Check sheet for the modelled part. Datum: model origin and axes. Units: mm. A direction names the side the tool comes from. Give positions to 0.01 mm unless a question says otherwise; leave off trailing zeros. Loops run counter-clockwise (first coordinate to the right, second up) from the corner with the lowest first, then second, coordinate; pieces in that order, holes last. Notation, with made-up numbers: (70, 38.25) - (119, 38.25) arc R20 ccw to (119, 64.25) - close; hole circle Ø3 at (50, 68.5). An arc over 180 degrees is marked (long way). Answer in a Markdown table with one row per item. Add a question column.
(1) Sectioned sample at D-D on y = 12.75. State how many separate pieces and enclosed holes the cut face has, then the cut area to 3 significant figures.
(2) Sectioned sample at C-C on x = -30.5. Enter the section's corners in (y, z).
(3) Thickness scan on L1, parallel to Z at x = 6.5, y = 11; L2, parallel to X at y = 14.25, z = 154.5; L3, parallel to Z at x = -19.5, y = 4. Record the ranges inside material, lowest first.
(4) Set-up check for faces 1 (the face through (0, 5, 128)), 2 (the face through (18.546, 10, 119)), 3 (the face through (8.945, 10.647, 149.074)), 4 (the face through (-0.31, 16.57, 128.29)): record each of +Z, -Z, +X, -X, +Y, -Y from which the full face is reachable in a straight line by a thin tool's end or side.
(5) Sectioned sample at A-A on x = 16. Enter the section's corners in (y, z).
(6) Draft check along Z on faces 5 (the face through (15.861, 11.11, 129.727)), 6 (the face through (29.046, 9.39, 161.315)), 7 (the face through (-22.925, 15, 143)). Enter one of: released by +Z, released by -Z, zero draft, split by the parting line, or undercut.
(7) Go/stop test with flat-tipped pins: P1, Ø1.5, axis at y = 11.5, z = 119.5, coming from the +X side; P2, Ø8, axis at x = -24, z = 135, coming from the +Y side; P3, Ø3, axis at y = 9.5, z = 135, coming from the +X side. Record where each tip stops, or that it passes through.
(8) Sectioned sample at B-B on z = 165. Enter the section's corners in (x, y), then the cut area to 3 significant figures.
from build123d import *

# Parameters (mm, degrees)
SKETCH2_W                       = 140.99708831
SKETCH2_H                       = 23.719356628
BOSS_EXTRUDE1_DEPTH             = 40
CUT_EXTRUDE1_DEPTH              = 229.787753821
BOSS_EXTRUDE2_DEPTH             = 16
CUT_EXTRUDE2_START              = -9
CUT_EXTRUDE2_DEPTH              = 9
FILLET1_R                       = 7
CUT_EXTRUDE3_DEPTH              = 194.183131235
CUT_EXTRUDE3_DEPTH_BACK         = 194.183131235
CUT_EXTRUDE4_DEPTH              = 194.497622924
BOSS_EXTRUDE4_REACH             = 195.183
SKETCH11_W                      = 140.99708831
SKETCH11_H                      = 8.5
BOSS_EXTRUDE4_DIRECTION_2_REACH = 195.183
SKETCH14_R                      = 0.7
CUT_EXTRUDE6_DEPTH              = 4
CUT_EXTRUDE7_DEPTH              = 202.370124673


with BuildPart() as part:
    # Sketch2 → Boss-Extrude1 (new body)
    with BuildSketch(Plane.XY.offset(138.608649029)):
        with Locations((-0.054079367, 11.859678314)):
            Rectangle(SKETCH2_W, SKETCH2_H)
    extrude(amount=BOSS_EXTRUDE1_DEPTH)

    # Sketch3 → Cut-Extrude1 (cut, through all)
    with BuildSketch(Plane.ZY.offset(70.552623522)):
        with BuildLine():
            Line((168.608649029, 23.719356628), (158.608649029, 23.719356628))
            Line((158.608649029, 23.719356628), (138.608649029, 23.719356628))
            Line((138.608649029, 23.719356628), (138.608649029, 5))
            ThreePointArc((138.608649029, 5), (156.289247948, 10.063699068), (168.608649029, 23.719356628))
        make_face()
    extrude(amount=-CUT_EXTRUDE1_DEPTH, mode=Mode.SUBTRACT)

    # Sketch4 → Boss-Extrude2 (add)
    with BuildSketch(Plane(origin=(0, 5, 0), x_dir=(1, 0, 0), z_dir=(0, 1, 0))):
        with BuildLine():
            Line((-22.924910668, -128.108649029), (-22.924910668, -168.608649029))
            Line((-22.924910668, -168.608649029), (-0.054079367, -168.608649029))
            Line((-0.054079367, -168.608649029), (22.816751934, -168.608649029))
            Line((22.816751934, -168.608649029), (22.816751934, -128.108649029))
            ThreePointArc((22.816751934, -128.108649029), (14.187021689, -127.958138772), (18.545920633, -120.508649029))
            Line((18.545920633, -120.508649029), (18.545920633, -117.508649029))
            Line((18.545920633, -117.508649029), (-18.654079367, -117.508649029))
            Line((-18.654079367, -117.508649029), (-18.654079367, -120.508649029))
            ThreePointArc((-18.654079367, -120.508649029), (-15.118545461, -121.973115123), (-13.654079367, -125.508649029))
            ThreePointArc((-13.654079367, -125.508649029), (-17.303923173, -130.322906838), (-22.924910668, -128.108649029))
        make_face()
    extrude(amount=BOSS_EXTRUDE2_DEPTH)

    # Sketch6 → Cut-Extrude2 (cut)
    with BuildSketch(Plane(origin=(0, 23.719356628, 0), x_dir=(1, 0, 0), z_dir=(0, 1, 0)).offset(CUT_EXTRUDE2_START)):
        with BuildLine():
            ThreePointArc((-18.654079367, -120.508649029), (-13.654079367, -125.508649029), (-18.654079367, -130.508649029))
            Line((-18.654079367, -130.508649029), (18.545920633, -130.508649029))
            ThreePointArc((18.545920633, -130.508649029), (13.545920633, -125.508649029), (18.545920633, -120.508649029))
            Line((18.545920633, -120.508649029), (18.545920633, -117.508649029))
            Line((18.545920633, -117.508649029), (-18.654079367, -117.508649029))
            Line((-18.654079367, -117.508649029), (-18.654079367, -120.508649029))
        make_face()
    extrude(amount=CUT_EXTRUDE2_DEPTH, mode=Mode.SUBTRACT)

    # Fillet1
    # the kernel refuses this fillet: 7 mm, written as the material it adds along each edge
    with BuildSketch(Plane(origin=(-36.061428038, 14.719356628, 130.508649029), x_dir=(0, 1, 0), z_dir=(1, 0, 0))) as fillet1_piece_1_section:
        with BuildLine():
            CenterArc((7, -6.962939469), FILLET1_R, 95.898427251, 84.101572749)
            Line((0, -6.962939469), (0, 0))
            Line((0, 0), (6.280643372, 0))
        make_face()
    fillet1_piece_1 = extrude(amount=72.014697343, mode=Mode.PRIVATE)
    fillet1_piece_1 = split(fillet1_piece_1, bisect_by=Plane(origin=(22.816751934, 16.511100944, 128.243610021), z_dir=(-1, 0, 0)), keep=Keep.TOP, mode=Mode.PRIVATE)
    fillet1_piece_1 = split(fillet1_piece_1, bisect_by=Plane(origin=(-22.924910668, 16.511100944, 128.243610021), z_dir=(1, 0, 0)), keep=Keep.TOP, mode=Mode.PRIVATE)
    fillet1_piece_1 = fillet1_piece_1 - Plane(origin=(18.545920633, 16.511100944, 125.508649029), x_dir=(0.854166260162501, 0, 0.5200000000000065), z_dir=(0, -1, 0)) * Cylinder(5, 172, mode=Mode.PRIVATE)
    fillet1_piece_1 = fillet1_piece_1 - Plane(origin=(-18.654079367, 16.511100944, 125.508649029), x_dir=(0, 0, -1), z_dir=(0, -1, 0)) * Cylinder(5, 172, mode=Mode.PRIVATE)
    add(fillet1_piece_1)

    # Sketch10 → Cut-Extrude3 (cut, two sides: drawn at the far end of the back side and taken through both)
    with BuildSketch(Plane(origin=(0, 21, 0), x_dir=(1, 0, 0), z_dir=(0, 1, 0)).offset(-CUT_EXTRUDE3_DEPTH_BACK)):
        with BuildLine():
            Line((-70.552623522, -168.608649029), (-70.552623522, -172.108649029))
            Line((-70.552623522, -172.108649029), (-56.424910668, -172.108649029))
            ThreePointArc((-56.424910668, -172.108649029), (-32.736833498, -162.296726199), (-22.924910668, -138.608649029))
            Line((-22.924910668, -138.608649029), (-70.552623522, -138.608649029))
            Line((-70.552623522, -138.608649029), (-70.552623522, -168.608649029))
        make_face()
        with BuildLine():
            ThreePointArc((22.816751934, -138.608649029), (32.628674764, -162.296726199), (56.316751934, -172.108649029))
            Line((56.316751934, -172.108649029), (70.444464788, -172.108649029))
            Line((70.444464788, -172.108649029), (70.444464788, -168.608649029))
            Line((70.444464788, -168.608649029), (70.444464788, -138.608649029))
            Line((70.444464788, -138.608649029), (22.816751934, -138.608649029))
        make_face()
    extrude(amount=CUT_EXTRUDE3_DEPTH + CUT_EXTRUDE3_DEPTH_BACK, mode=Mode.SUBTRACT)

    # Sketch12 → Cut-Extrude4 (cut, through all)
    with BuildSketch(Plane(origin=(0, 23.719356628, 0), x_dir=(1, 0, 0), z_dir=(0, 1, 0))):
        with BuildLine():
            ThreePointArc((39.183618102, -173.086260969), (47.517265008, -176.089564571), (56.316751934, -177.108649029))
            Line((56.316751934, -177.108649029), (70.444464788, -177.108649029))
            Line((70.444464788, -177.108649029), (70.444464788, -172.108649029))
            Line((70.444464788, -172.108649029), (56.316751934, -172.108649029))
            ThreePointArc((56.316751934, -172.108649029), (32.628674764, -162.296726199), (22.816751934, -138.608649029))
            ThreePointArc((22.816751934, -138.608649029), (27.116175744, -157.691232929), (39.183618102, -173.086260969))
        make_face()
        with BuildLine():
            Line((-70.552623522, -172.108649029), (-70.552623522, -177.108649029))
            Line((-70.552623522, -177.108649029), (-56.424910668, -177.108649029))
            ThreePointArc((-56.424910668, -177.108649029), (-47.625423742, -176.089564571), (-39.291776836, -173.086260969))
            ThreePointArc((-39.291776836, -173.086260969), (-27.224334478, -157.691232929), (-22.924910668, -138.608649029))
            ThreePointArc((-22.924910668, -138.608649029), (-32.736833498, -162.296726199), (-56.424910668, -172.108649029))
            Line((-56.424910668, -172.108649029), (-70.552623522, -172.108649029))
        make_face()
    extrude(amount=-CUT_EXTRUDE4_DEPTH, mode=Mode.SUBTRACT)

    # Boss-Extrude4: up to this face of the body (flat: up to its plane)
    boss_extrude4_end = Plane(part.part.faces().sort_by_distance((-0.054079367, 23.719356628, 174.251451193))[0])
    # Sketch11 → Boss-Extrude4 (add, up to the picked face)
    with BuildSketch(Plane(origin=(0, 21, 0), x_dir=(1, 0, 0), z_dir=(0, 1, 0)), mode=Mode.PRIVATE) as boss_extrude4_sk1:
        with Locations((-0.054079367, -182.858649029)):
            Rectangle(SKETCH11_W, SKETCH11_H)
    boss_extrude4_tool1 = split(extrude(boss_extrude4_sk1.sketch, amount=BOSS_EXTRUDE4_REACH, mode=Mode.PRIVATE), bisect_by=boss_extrude4_end, keep=Keep.BOTH, mode=Mode.PRIVATE)
    add(boss_extrude4_tool1.solids().sort_by(Axis((-0.054079, 21, 182.858649), (0, 1, 0)))[0])

    # Boss-Extrude4 direction 2: up to this face of the body (flat: up to its plane)
    boss_extrude4_direction_2_end = Plane(part.part.faces().sort_by_distance((-0.054079367, 0, 161.750198619))[0])
    # Sketch11 → Boss-Extrude4 direction 2 (add, up to the picked face)
    with BuildSketch(Plane(origin=(0, 21, 0), x_dir=(1, 0, 0), z_dir=(0, 1, 0)), mode=Mode.PRIVATE) as boss_extrude4_direction_2_sk1:
        with Locations((-0.054079367, -182.858649029)):
            Rectangle(SKETCH11_W, SKETCH11_H)
    boss_extrude4_direction_2_tool1 = split(extrude(boss_extrude4_direction_2_sk1.sketch, amount=-BOSS_EXTRUDE4_DIRECTION_2_REACH, mode=Mode.PRIVATE), bisect_by=boss_extrude4_direction_2_end, keep=Keep.BOTH, mode=Mode.PRIVATE)
    add(boss_extrude4_direction_2_tool1.solids().sort_by(Axis((-0.054079, 21, 182.858649), (0, -1, 0)))[0])

    # Sketch14 → Cut-Extrude6 (cut)
    with BuildSketch(Plane(origin=(0, 21, 0), x_dir=(1, 0, 0), z_dir=(0, 1, 0))):
        with Locations(Location((-10.054079367, -162.11771624, 0), (0, 0, 270))):
            Circle(SKETCH14_R)
        with Locations(Location((9.945920633, -162.11771624, 0), (0, 0, 90))):
            Circle(SKETCH14_R)
    extrude(amount=-CUT_EXTRUDE6_DEPTH, mode=Mode.SUBTRACT)

    # Sketch16 → Cut-Extrude7 (cut, through all)
    with BuildSketch(Plane(origin=(0, 23.719356628, 0), x_dir=(1, 0, 0), z_dir=(0, 1, 0))):
        with BuildLine():
            Line((-7.054079367, -151.11771624), (-5.054079367, -151.11771624))
            ThreePointArc((-5.054079367, -151.11771624), (-3.054079367, -149.11771624), (-5.054079367, -147.11771624))
            Line((-5.054079367, -147.11771624), (-7.054079367, -147.11771624))
            ThreePointArc((-7.054079367, -147.11771624), (-9.054079367, -149.11771624), (-7.054079367, -151.11771624))
        make_face()
        with BuildLine():
            ThreePointArc((4.945920633, -151.11771624), (2.945920633, -149.11771624), (4.945920633, -147.11771624))
            Line((4.945920633, -147.11771624), (6.945920633, -147.11771624))
            ThreePointArc((6.945920633, -147.11771624), (8.945920633, -149.11771624), (6.945920633, -151.11771624))
            Line((6.945920633, -151.11771624), (4.945920633, -151.11771624))
        make_face()
        with BuildLine():
            Line((4.945920633, -171.11771624), (6.945920633, -171.11771624))
            ThreePointArc((6.945920633, -171.11771624), (8.529924172, -170.338753827), (8.880048492, -168.608649029))
            Line((8.880048492, -168.608649029), (3.011792774, -168.608649029))
            ThreePointArc((3.011792774, -168.608649029), (3.361917094, -170.338753827), (4.945920633, -171.11771624))
        make_face()
        with BuildLine():
            Line((3.011792774, -168.608649029), (8.880048492, -168.608649029))
            ThreePointArc((8.880048492, -168.608649029), (8.16695822, -167.533712701), (6.945920633, -167.11771624))
            Line((6.945920633, -167.11771624), (4.945920633, -167.11771624))
            ThreePointArc((4.945920633, -167.11771624), (3.724883046, -167.533712701), (3.011792774, -168.608649029))
        make_face()
        with BuildLine():
            Line((-8.988207226, -168.608649029), (-3.119951508, -168.608649029))
            ThreePointArc((-3.119951508, -168.608649029), (-3.83304178, -167.533712701), (-5.054079367, -167.11771624))
            Line((-5.054079367, -167.11771624), (-7.054079367, -167.11771624))
            ThreePointArc((-7.054079367, -167.11771624), (-8.275116954, -167.533712701), (-8.988207226, -168.608649029))
        make_face()
        with BuildLine():
            ThreePointArc((-5.054079367, -171.11771624), (-3.470075828, -170.338753827), (-3.119951508, -168.608649029))
            Line((-3.119951508, -168.608649029), (-8.988207226, -168.608649029))
            ThreePointArc((-8.988207226, -168.608649029), (-8.638082906, -170.338753827), (-7.054079367, -171.11771624))
            Line((-7.054079367, -171.11771624), (-5.054079367, -171.11771624))
        make_face()
    extrude(amount=-CUT_EXTRUDE7_DEPTH, mode=Mode.SUBTRACT)


solid = part.part
Reply:
| question | item | result |
|---|---|---|
| 1 | separate pieces | 1 |
| 1 | enclosed holes | 4 |
| 1 | area | 4,310 mm^2 |
| 2 | outline | (0, 163.44) - (16.07, 163.44) arc R33.4 cw to (23.72, 168.61) - (23.72, 187.11) - (0, 187.11) - close |
| 3 | L1 | 117.51 to 147.12, 151.12 to 167.12, 171.12 to 187.11 |
| 3 | L2 | -22.92 to 22.82 |
| 3 | L3 | 138.61 to 187.11 |
| 4 | face 1 | -Z, +X, -X, -Y |
| 4 | face 2 | -Z, +X, +Y, -Y |
| 4 | face 3 | +Y, -Y |
| 4 | face 4 | -Z, +Y |
| 5 | outline | (0, 138.61) - (5, 138.61) - (5, 129.81) - (18.6, 129.81) arc R7 cw to (21, 130.51) - (21, 167.12) arc R33.4 cw to (23.72, 168.61) - (23.72, 187.11) - (0, 187.11) - close; (5, 117.51) - (14.72, 117.51) - (14.72, 121.21) - (5, 121.21) - close |
| 6 | face 5 | undercut |
| 6 | face 6 | released by -Z |
| 6 | face 7 | zero draft |
| 7 | P1 | x = 18.55 |
| 7 | P2 | y = 21 |
| 7 | P3 | x = 22.82 |
| 8 | outline | (-31.6, 0) - (31.49, 0) - (31.49, 17.93) - (22.82, 17.93) - (22.82, 21) - (-22.92, 21) - (-22.92, 17.93) - (-31.6, 17.93) - close |
| 8 | area | 1,270 mm^2 |
